Solid Edge part; units mm, degrees
sketch "Sketch1" plane through (0, 0, 0) normal (0, -1, 0) x (1, 0, 0)
  circle A0 centre (0, 0) radius 93.05
  circle A1 centre (0, 0) radius 16.25
extrude "Protrusion1" add sketch "Sketch1" against normal blind 3
hole "Hole_1" at (0, 0, 32) direction (0, 1, 0) diameter 8 end up to next
pattern_circular "Pattern2" count 4 over 360 about axis through (0, 0, 0) along (0, 1, 0) of "Hole_1"
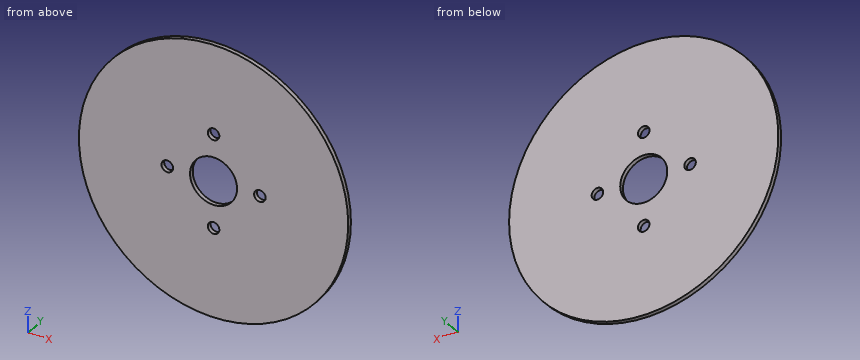
The model under review builds one solid part; all positions refer to its coordinate system, in mm. Round coordinates to 2 decimals unless told otherwise and drop trailing zeros. Write each loop counter-clockwise with the first axis right and the second up, starting at its lowest first coordinate (ties: lowest second). Pieces come first, ordered by that corner, then holes.
(1) We need section B-B on z = 0. Give the boundary of the cut face in (x, y).
(2) Insertion check: pin 1 (1.5 mm diameter, centred on y = 1, z = 32.5, fed in from +X); pin 2 (7 mm diameter, centred on x = 0, z = -32, fed in from +Y); pin 3 (1.5 mm diameter, centred on y = 2.5, z = -32, fed in from -X); pin 4 (1.5 mm diameter, centred on x = 48, y = 2.5, fed in from +Z). Each pin has a flat end and moves straight along its axis. Give the tip position at first contact, or say it passes through.
(3) We need section C-C on y = 2.1. Give the boundary of the cut face in (x, z).
(4) Wall thickness on L1, parallel to Z at x = 0, y = 1.6; L2, parallel to X at y = 1.35, z = -32; L3, parallel to X at y = 1.65, z = -33: over which ranges is each line inside the solid? List them lowest first.
(5) We need section A-A on x = 0. Give the boundary of the cut face in (y, z).
(6) We need section D-D on x = -32. Give the boundary of the cut face in (y, z).
Findings below:
1. outline: (-93.05, 0) - (-36, 0) - (-36, 3) - (-93.05, 3) - close; (-28, 0) - (-16.25, 0) - (-16.25, 3) - (-28, 3) - close; (16.25, 0) - (28, 0) - (28, 3) - (16.25, 3) - close; (36, 0) - (93.05, 0) - (93.05, 3) - (36, 3) - close
2. pin 1: stops at x = 87.47
2. pin 2: passes through
2. pin 3: stops at x = -87.65
2. pin 4: stops at z = 80.16
3. outline: circle Ø186.1 at (0, 0); hole circle Ø8 at (-32, 0); hole circle Ø32.5 at (0, 0); hole circle Ø8 at (0, -32); hole circle Ø8 at (0, 32); hole circle Ø8 at (32, 0)
4. L1: z = -93.05 to -36, -28 to -16.25, 16.25 to 28, 36 to 93.05
4. L2: x = -87.37 to -4, 4 to 87.37
4. L3: x = -87 to -3.87, 3.87 to 87
5. outline: (0, -93.05) - (3, -93.05) - (3, -36) - (0, -36) - close; (0, -28) - (3, -28) - (3, -16.25) - (0, -16.25) - close; (0, 16.25) - (3, 16.25) - (3, 28) - (0, 28) - close; (0, 36) - (3, 36) - (3, 93.05) - (0, 93.05) - close
6. outline: (0, -87.37) - (3, -87.37) - (3, -4) - (0, -4) - close; (0, 4) - (3, 4) - (3, 87.37) - (0, 87.37) - close
